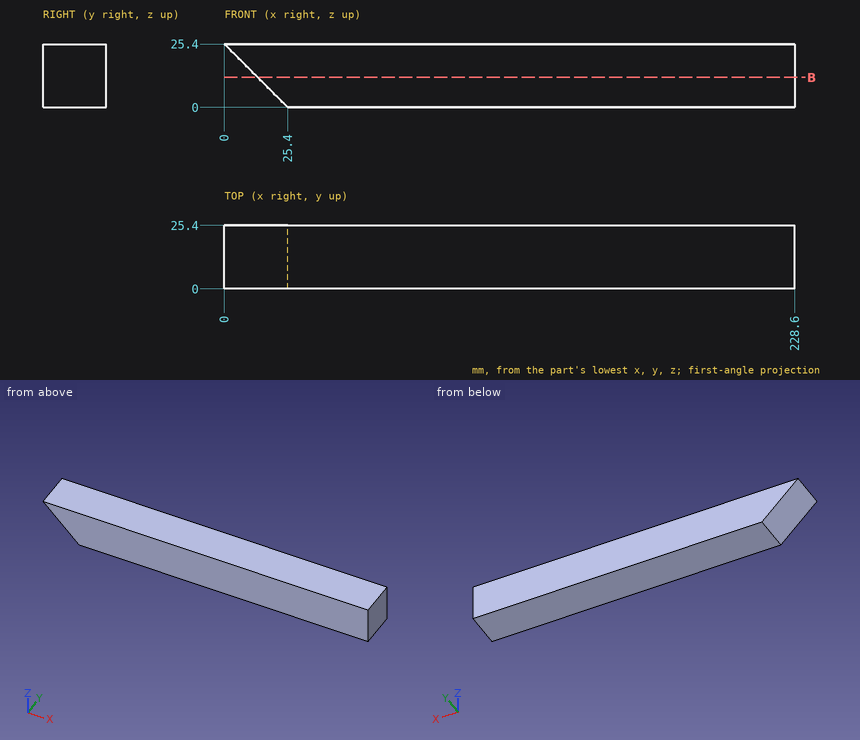
Design review of the part shown in the three views and the two pictorial views. Dimensions are in mm from the part's minimum x, y and z. Round coordinates to 2 decimals unless told otherwise and drop trailing zeros. Write each loop counter-clockwise with the first axis right and the second up, starting at its lowest first coordinate (ties: lowest second). Pieces come first, ordered by that corner, then holes. Notation, with made-up numbers: (59.25, -30) -> (67.25, -30) arc R14 ccw to (67.25, -23) -> close; hole circle Ø4 at (17.25, 65.25). An arc over 180 degrees is marked (long way). One line per question, with ' | ' between items. Start each with the question number.
1) For pin 1 Ø6 at (y, z) = (17, 14.5) entering from -X, flat-tipped, find the tip position at first contact; note if it passes through.
2) Add section B-B (z = 12). Write out the cut boundary in (x, y), and give its area (3 significant figures).
3) Wall thickness on line 1 along X through (y, z) = (18, 17.5); line 2 along Z through (x, y) = (24, 21); line 3 along X through (y, z) = (18.25, 17): over which ranges is each line inside the solid? List them lowest first.
Reported:
1) pin 1: stops at x = 7.9
2) outline: (13.4, 0) -> (228.6, 0) -> (228.6, 25.4) -> (13.4, 25.4) -> close | area: 5,470 mm²
3) line 1: x = 7.9 to 228.6 | line 2: z = 1.4 to 25.4 | line 3: x = 8.4 to 228.6
